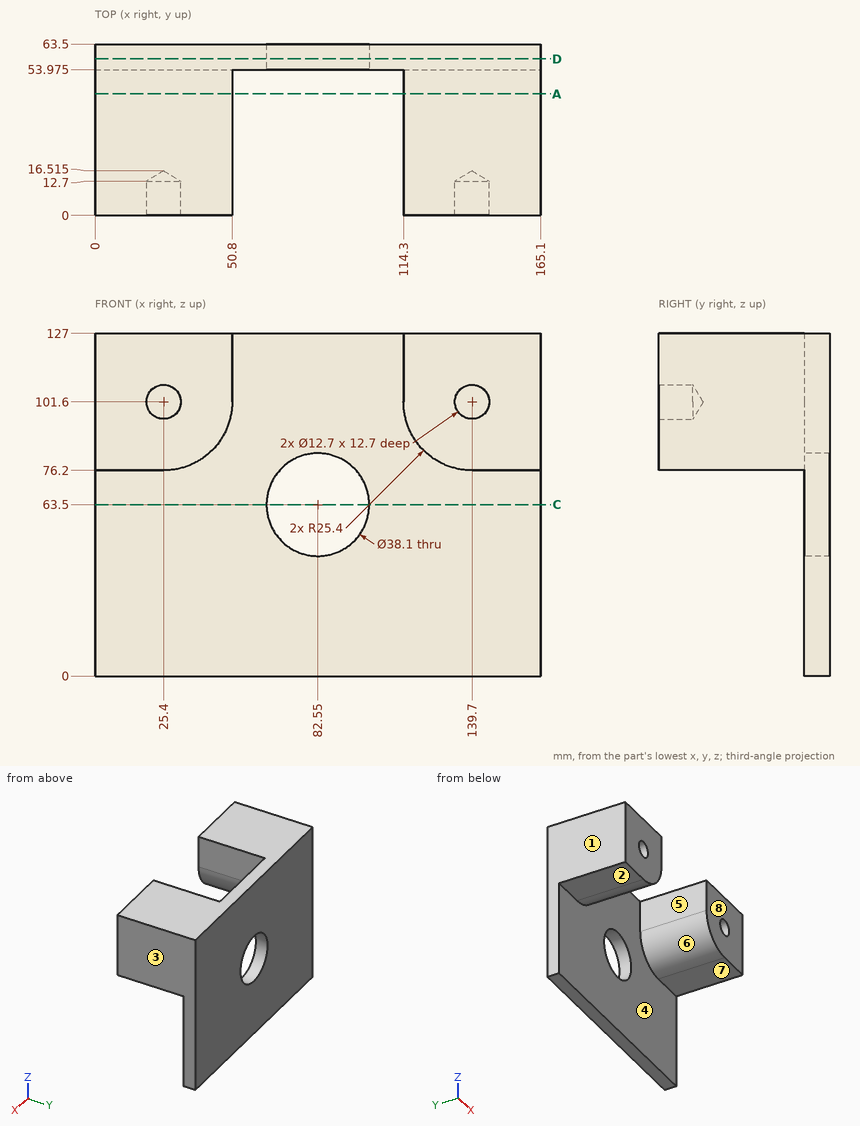
Job drawing, mm, ordinate dimensions from the low corner. One solid piece. A direction names the side the tool comes from. Round coordinates to 2 decimals unless told otherwise and drop trailing zeros. Loops run counter-clockwise (first coordinate to the right, second up) from the corner with the lowest first, then second, coordinate; pieces in that order, holes last.
(1) Cut at A-A (y = 45). Give the cut face in (x, z), plus the area to 3 significant figures.
(2) Cut at D-D (y = 58). Give the cut face in (x, z).
(3) Wall check: line 1 along X through (y, z) = (38.5, 101); line 2 along Z through (x, y) = (82.55, 56.75); line 3 along Z through (x, y) = (139.7, 3.5). Give the ranges that are in metal, low to high.
(4) Cut at C-C (z = 63.5). Give the cut face in (x, y) (1 decimal), plus the area to 3 significant figures.
(5) Two-plate mould, pull along X, no slides. Class the marked faces 1, 2, 3 and 4: +X half, -X half, draft (parallel to the pull), parting line (faces both ways), or undercut.
(6) Which spindle directions (+Z, -Z, +X, -X, +Y, -Y) get a long thin tool onto all of the face, cutting with end or side? Do the marked faces 5, 6, 7 and 8. Say none if no direction does.
(7) Drop flat-ended pins along their axis: pin 1 (12 mm diameter, centred on x = 34.5, y = 46, fed in from -Z); pin 2 (7.5 mm diameter, centred on x = 11, y = 25.5, fed in from -Z); pin 3 (10 mm diameter, centred on y = 44, z = 76, fed in from -X); pin 4 (2 mm diameter, centred on x = 119, y = 18, fed in from -Z) (1 decimal). Give the stop position or say it passes through.
Findings below:
1. outline: (0, 76.2) - (25.4, 76.2) arc R25.4 ccw to (50.8, 101.6) - (50.8, 127) - (0, 127) - close; (114.3, 101.6) arc R25.4 ccw to (139.7, 76.2) - (165.1, 76.2) - (165.1, 127) - (114.3, 127) - close
1. area: 4,880 mm2
2. outline: (0, 0) - (165.1, 0) - (165.1, 127) - (0, 127) - close; hole circle Ø38.1 at (82.55, 63.5)
3. line 1: x = 0 to 50.79, 114.31 to 165.1
3. line 2: z = 0 to 44.45, 82.55 to 127
3. line 3: z = 76.2 to 95.25, 107.95 to 127
4. outline: (0, 54) - (63.5, 54) - (63.5, 63.5) - (0, 63.5) - close; (101.6, 54) - (165.1, 54) - (165.1, 63.5) - (101.6, 63.5) - close
4. area: 1,210 mm2
5. face 1: -X half
5. face 2: draft
5. face 3: +X half
5. face 4: undercut
6. face 5: +Z, -Z, -Y
6. face 6: -Z, -Y
6. face 7: -Z, +X, -X, -Y
6. face 8: +Z, -Z, +X, -X, -Y
7. pin 1: stops at z = 76.39
7. pin 2: stops at z = 76.2
7. pin 3: stops at x = 0
7. pin 4: stops at z = 85.6
